```python
from build123d import *

# Parameters (mm, degrees)
CYLINDER065_R     = 2.6
CYLINDER065_DEPTH = 2
CYLINDER064_R     = 2.5
CYLINDER064_DEPTH = 5


with BuildPart() as cilindro065:
    # Cylinder065 → Cylinder065 (new body)
    with BuildSketch(Plane.XY.offset(5)):
        Circle(CYLINDER065_R)
    extrude(amount=CYLINDER065_DEPTH)


with BuildPart() as obj1:
    # Cylinder064 → Cylinder064 (new body)
    with BuildSketch(Plane.XY):
        Circle(CYLINDER064_R)
    extrude(amount=CYLINDER064_DEPTH)

    # Fusion022: union Cilindro065
    add(cilindro065.part)


solid = obj1.part
```
Can you work these out from the model? Positions are in its coordinate system, mm. Round coordinates to 2 decimals unless told otherwise and drop trailing zeros. Loops run counter-clockwise (first coordinate to the right, second up) from the corner with the lowest first, then second, coordinate; pieces in that order, holes last.
Item 1: Suppose I cut it at C-C, the plane z = 4.5. Write out the boundary of the cut face in (x, y).
Item 2: Please list where these lines run through material, in increasing order: L1, parallel to Y at x = 0, z = 0.75; L2, parallel to X at y = -0.1, z = 6; L3, parallel to X at y = -1.35, z = 1.25.
Item 3: Will these pins go through, and if not, where does the flat tip stop? pin 1 Ø3 at (x, z) = (0, 2.5) entering from -Y; pin 2 Ø1.5 at (x, z) = (0, 4) entering from +Y.
Item 4: Suppose I cut it at A-A, the plane y = 0. Write out the boundary of the cut face in (x, z), then the cut area to 3 significant figures.
Item 5: If we mould it in two halves opening along Z, with no side actions, what happens to faces 1 (the flat face through (0, 0, 0)), 2 (the flat face through (0, 0, 7)), 3 (the cylindrical face through (-0.54, -2.44, 2.46))? For each: +Z half, -Z half, draft (parallel to the pull), parting line (faces both ways), or undercut.
Item 6: Suppose I cut it at D-D, the plane z = 5.5. Write out the boundary of the cut face in (x, y).
Reported:
1. outline: circle Ø5 at (0, 0)
2. L1: y = -2.5 to 2.5
2. L2: x = -2.6 to 2.6
2. L3: x = -2.1 to 2.1
3. pin 1: stops at y = -2.5
3. pin 2: stops at y = 2.5
4. outline: (-2.6, 5) - (-2.5, 5) - (-2.5, 0) - (2.5, 0) - (2.5, 5) - (2.6, 5) - (2.6, 7) - (-2.6, 7) - close
4. area: 35.4 mm2
5. face 1: -Z half
5. face 2: +Z half
5. face 3: draft
6. outline: circle Ø5.2 at (0, 0)
